Read the model definition and answer for the solid it produces. Units are mm, in the model's axes. Face numbers are marked on the shaded views. Give positions to 0.01 mm unless a question says otherwise; leave off trailing zeros. Use a Markdown table: item, result. Add a question column.
Item 1: Consider probe 1 along X at (y, z) = (22.7, 0); probe 2 along X at (y, z) = (22.7, 68); probe 3 along Y at (x, z) = (63.5, -25). Determine where each line is inside the solid, lowest interval first. Write a range as [from, to].
Item 2: The mould has two halves that part along Z. Classify the marked faces 1 and 2: pulls with the +Z half, pulls with the -Z half, needs draft (parallel to the pull), parting line crosses it, or undercut.
Item 3: Given P1, Ø2, axis at x = 5.5, y = 15, coming from the +Z side; P2, Ø6, axis at x = 0, z = 68, coming from the +Y side; P3, Ø5, axis at x = 2, z = 67.5, coming from the -Y side, each flat-ended and moving along its own axis, determine where each tip first touches the part or whether it passes through.
from build123d import *

# Parameters (mm, degrees)
BOSS_EXTRUDE1_REACH            = 121.943
SKETCH2_R                      = 2
CUT_EXTRUDE1_REACH             = 123.084
SKETCH4_W                      = 180
SKETCH4_H                      = 15
CUT_EXTRUDE1_DIRECTION_2_REACH = 123.084
SKETCH5_R                      = 74.701116641
SKETCH5_R_2                    = 2
BOSS_EXTRUDE2_DEPTH            = 2
SKETCH6_R                      = 5
CUT_EXTRUDE2_DEPTH             = 8
FILLET1_R                      = 2
FILLET2_R                      = 10
CUT_EXTRUDE3_REACH             = 120.264


with BuildPart() as part:
    # Sketch1 → Revolve-Thin1 (revolve)
    with BuildSketch(Plane.XY, mode=Mode.PRIVATE) as revolve_thin1_sk:
        with BuildLine():
            ThreePointArc((-70, 0), (-72.962243847, 16.05699404), (-81.458980338, 30))
            Line((-81.458980338, 30), (-82.949692323, 28.666666667))
            ThreePointArc((-82.949692323, 28.666666667), (-74.830588565, 15.34334986), (-72, 0))
            Line((-72, 0), (-70, 0))
        make_face()
    revolve(revolve_thin1_sk.sketch.rotate(Axis((0, 0, 0), (0, 1, 0)), 270), axis=Axis((0, 0, 0), (0, 1, 0)))

    # Boss-Extrude1: up to this face of the body (flat: up to its plane)
    boss_extrude1_end = Plane(part.part.faces().sort_by_distance((0, 0, 71.796353247))[0])
    # Sketch2 → Boss-Extrude1 (add, up to the picked face)
    with BuildSketch(Plane(origin=(0, 25, 0), x_dir=(-1, 0, 0), z_dir=(0, -1, 0)), mode=Mode.PRIVATE) as boss_extrude1_sk1:
        with BuildLine():
            ThreePointArc((6.495313924, -70.609769534), (4.324225171, -78.519680843), (4, -86.715728753))
            Line((4, -86.715728753), (-4, -86.715728753))
            ThreePointArc((-4, -86.715728753), (-4.324225171, -78.519680843), (-6.495313924, -70.609769534))
            ThreePointArc((-6.495313924, -70.609769534), (0, -61), (6.495313924, -70.609769534))
        make_face()
        with Locations(Location((0, -68, 0), (0, 0, 90))):
            Circle(SKETCH2_R, mode=Mode.SUBTRACT)
    boss_extrude1_tool1 = split(extrude(boss_extrude1_sk1.sketch, amount=BOSS_EXTRUDE1_REACH, mode=Mode.PRIVATE), bisect_by=boss_extrude1_end, keep=Keep.BOTH, mode=Mode.PRIVATE)
    # Sketch2 → Boss-Extrude1 (add, up to the picked face)
    with BuildSketch(Plane(origin=(0, 25, 0), x_dir=(-1, 0, 0), z_dir=(0, -1, 0)), mode=Mode.PRIVATE) as boss_extrude1_sk2:
        with BuildLine():
            ThreePointArc((70.609769534, 6.495313924), (78.519680843, 4.324225171), (86.715728753, 4))
            Line((86.715728753, 4), (86.715728753, -4))
            ThreePointArc((86.715728753, -4), (78.519680843, -4.324225171), (70.609769534, -6.495313924))
            ThreePointArc((70.609769534, -6.495313924), (61, 0), (70.609769534, 6.495313924))
        make_face()
        with Locations(Location((68, 0, 0), (0, 0, 90))):
            Circle(SKETCH2_R, mode=Mode.SUBTRACT)
    boss_extrude1_tool2 = split(extrude(boss_extrude1_sk2.sketch, amount=BOSS_EXTRUDE1_REACH, mode=Mode.PRIVATE), bisect_by=boss_extrude1_end, keep=Keep.BOTH, mode=Mode.PRIVATE)
    # Sketch2 → Boss-Extrude1 (add, up to the picked face)
    with BuildSketch(Plane(origin=(0, 25, 0), x_dir=(-1, 0, 0), z_dir=(0, -1, 0)), mode=Mode.PRIVATE) as boss_extrude1_sk3:
        with BuildLine():
            ThreePointArc((-6.495313924, 70.609769534), (-4.324225171, 78.519680843), (-4, 86.715728753))
            Line((-4, 86.715728753), (4, 86.715728753))
            ThreePointArc((4, 86.715728753), (4.324225171, 78.519680843), (6.495313924, 70.609769534))
            ThreePointArc((6.495313924, 70.609769534), (0, 61), (-6.495313924, 70.609769534))
        make_face()
        with Locations(Location((0, 68, 0), (0, 0, 90))):
            Circle(SKETCH2_R, mode=Mode.SUBTRACT)
    boss_extrude1_tool3 = split(extrude(boss_extrude1_sk3.sketch, amount=BOSS_EXTRUDE1_REACH, mode=Mode.PRIVATE), bisect_by=boss_extrude1_end, keep=Keep.BOTH, mode=Mode.PRIVATE)
    # Sketch2 → Boss-Extrude1 (add, up to the picked face)
    with BuildSketch(Plane(origin=(0, 25, 0), x_dir=(-1, 0, 0), z_dir=(0, -1, 0)), mode=Mode.PRIVATE) as boss_extrude1_sk4:
        with BuildLine():
            ThreePointArc((-81.360361137, 4.007132799), (-81.434321805, 2.004173085), (-81.458980338, 0))
            ThreePointArc((-81.458980338, 0), (-81.434321805, -2.004173085), (-81.360361137, -4.007132799))
            ThreePointArc((-81.360361137, -4.007132799), (-75.887045081, -4.837355971), (-70.605732867, -6.496934371))
            ThreePointArc((-70.605732867, -6.496934371), (-61, 0), (-70.605732867, 6.496934371))
            ThreePointArc((-70.605732867, 6.496934371), (-75.887045081, 4.837355971), (-81.360361137, 4.007132799))
        make_face()
        with Locations(Location((-68, 0, 0), (0, 0, 90))):
            Circle(SKETCH2_R, mode=Mode.SUBTRACT)
    boss_extrude1_tool4 = split(extrude(boss_extrude1_sk4.sketch, amount=BOSS_EXTRUDE1_REACH, mode=Mode.PRIVATE), bisect_by=boss_extrude1_end, keep=Keep.BOTH, mode=Mode.PRIVATE)
    add(boss_extrude1_tool1.solids().sort_by(Axis((0, 25, 73.20964), (0, -1, 0)))[0])
    add(boss_extrude1_tool2.solids().sort_by(Axis((-73.20964, 25, 0), (0, -1, 0)))[0])
    add(boss_extrude1_tool3.solids().sort_by(Axis((0, 25, -73.20964), (0, -1, 0)))[0])
    add(boss_extrude1_tool4.solids().sort_by(Axis((71.031369, 25, 0), (0, -1, 0)))[0])

    # Sketch3 → Cut-Revolve1 (revolve, cut)
    with BuildSketch(Plane.XY, mode=Mode.PRIVATE) as cut_revolve1_sk:
        with BuildLine():
            Line((-72, 0), (-99.127196695, 0))
            Line((-99.127196695, 0), (-99.127196695, 28.666666667))
            Line((-99.127196695, 28.666666667), (-82.949692323, 28.666666667))
            ThreePointArc((-82.949692323, 28.666666667), (-74.830588565, 15.34334986), (-72, 0))
        make_face()
    revolve(cut_revolve1_sk.sketch.rotate(Axis((0, 0, 0), (0, 1, 0)), 270), axis=Axis((0, 0, 0), (0, 1, 0)), mode=Mode.SUBTRACT)

    # Sketch4 → Cut-Extrude1 (cut, up to next)
    with BuildSketch(Plane(origin=(0, 0, 0), x_dir=(0, 0, -1), z_dir=(1, 0, 0)), mode=Mode.PRIVATE) as cut_extrude1_sk1:
        with Locations((0, 7.5)):
            Rectangle(SKETCH4_W, SKETCH4_H)
    cut_extrude1_tool1 = extrude(cut_extrude1_sk1.sketch, amount=-CUT_EXTRUDE1_REACH, mode=Mode.PRIVATE) & part.part
    add(cut_extrude1_tool1.solids().sort_by_distance((0, 7.5, 0))[0], mode=Mode.SUBTRACT)

    # Sketch4 → Cut-Extrude1 direction 2 (cut, up to next)
    with BuildSketch(Plane(origin=(0, 0, 0), x_dir=(0, 0, -1), z_dir=(1, 0, 0)), mode=Mode.PRIVATE) as cut_extrude1_direction_2_sk1:
        with Locations((0, 7.5)):
            Rectangle(SKETCH4_W, SKETCH4_H)
    cut_extrude1_direction_2_tool1 = extrude(cut_extrude1_direction_2_sk1.sketch, amount=CUT_EXTRUDE1_DIRECTION_2_REACH, mode=Mode.PRIVATE) & part.part
    add(cut_extrude1_direction_2_tool1.solids().sort_by_distance((0, 7.5, 0))[0], mode=Mode.SUBTRACT)

    # Sketch5 → Boss-Extrude2 (add)
    with BuildSketch(Plane.XZ.offset(-15)):
        with Locations(Location((0, 0, 0), (0, 0, 270))):
            Circle(SKETCH5_R)
        with Locations(Location((68, 0, 0), (0, 0, 270))):
            Circle(SKETCH5_R_2, mode=Mode.SUBTRACT)
        with Locations(Location((0, 68, 0), (0, 0, 270))):
            Circle(SKETCH5_R_2, mode=Mode.SUBTRACT)
        with Locations(Location((-68, 0, 0), (0, 0, 270))):
            Circle(SKETCH5_R_2, mode=Mode.SUBTRACT)
        with Locations(Location((0, -68, 0), (0, 0, 270))):
            Circle(SKETCH5_R_2, mode=Mode.SUBTRACT)
    extrude(amount=BOSS_EXTRUDE2_DEPTH)

    # Sketch6 → Cut-Extrude2 (cut)
    with BuildSketch(Plane.XZ.offset(-13)):
        with Locations(Location((0, 68, 0), (0, 0, 270))):
            Circle(SKETCH6_R)
        with Locations(Location((68, 0, 0), (0, 0, 270))):
            Circle(SKETCH6_R)
        with Locations(Location((0, -68, 0), (0, 0, 270))):
            Circle(SKETCH6_R)
        with Locations(Location((-68, 0, 0), (0, 0, 270))):
            Circle(SKETCH6_R)
    extrude(amount=-CUT_EXTRUDE2_DEPTH, mode=Mode.SUBTRACT)

    # Fillet1
    # the kernel refuses this fillet: 2 mm, written as the material it takes off along each edge
    with BuildSketch(Plane(origin=(0, 13, 0), x_dir=(0, 0, -1), z_dir=(-1, 0, 0))) as fillet1_piece_1:
        with BuildLine():
            CenterArc((74.701116641 - FILLET1_R, -FILLET1_R), FILLET1_R, 0, 90)
            Line((74.701116641 - FILLET1_R, 0), (74.701116641, 0))
            Line((74.701116641, 0), (74.701116641, -FILLET1_R))
        make_face()
    revolve(axis=Axis((0, 13, 0), (0, -1, 0)), mode=Mode.SUBTRACT)

    # Fillet2
    fillet2_edges = [part.edges().sort_by_distance(p)[0] for p in [
        (0, 15, 74.701116641),
    ]]
    fillet(fillet2_edges, radius=FILLET2_R)

    # Sketch7 → Cut-Extrude3 (cut, up to next)
    with BuildSketch(Plane(origin=(0, 15, 0), x_dir=(1, 0, 0), z_dir=(0, 1, 0)), mode=Mode.PRIVATE) as cut_extrude3_sk1:
        with BuildLine():
            Line((10.606601718, -31.819805153), (31.819805153, -10.606601718))
            ThreePointArc((31.819805153, -10.606601718), (34.748737342, -3.535533906), (31.819805153, 3.535533906))
            Line((31.819805153, 3.535533906), (3.535533906, 31.819805153))
            ThreePointArc((3.535533906, 31.819805153), (-3.535533906, 34.748737342), (-10.606601718, 31.819805153))
            Line((-10.606601718, 31.819805153), (-31.819805153, 10.606601718))
            ThreePointArc((-31.819805153, 10.606601718), (-34.748737342, 3.535533906), (-31.819805153, -3.535533906))
            Line((-31.819805153, -3.535533906), (-3.535533906, -31.819805153))
            ThreePointArc((-3.535533906, -31.819805153), (3.535533906, -34.748737342), (10.606601718, -31.819805153))
        make_face()
    cut_extrude3_tool1 = extrude(cut_extrude3_sk1.sketch, amount=-CUT_EXTRUDE3_REACH, mode=Mode.PRIVATE) & part.part
    add(cut_extrude3_tool1.solids().sort_by_distance((0, 15, 0))[0], mode=Mode.SUBTRACT)


solid = part.part
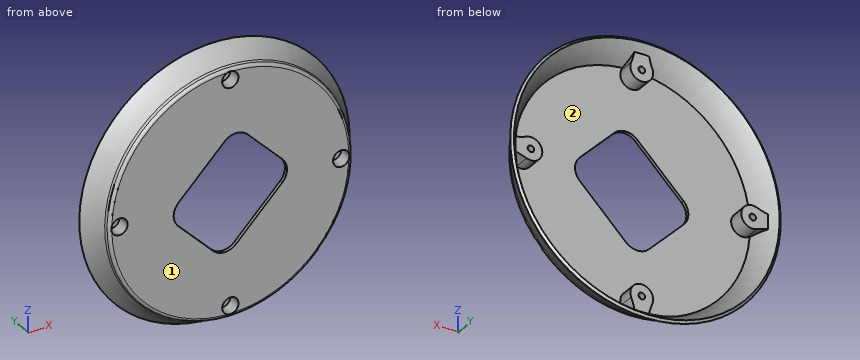
Filled in:
| question | item | result |
|---|---|---|
| 1 | probe 1 | [-78.48, -70], [-66, -61], [61, 66], [70, 78.48] |
| 1 | probe 2 | [-39.18, -34.26], [-7, -2], [2, 7], [34.26, 39.18] |
| 1 | probe 3 | [13, 15] |
| 2 | face 1 | needs draft |
| 2 | face 2 | undercut |
| 3 | P1 | z = 74.89 |
| 3 | P2 | y = 25 |
| 3 | P3 | y = 21 |
